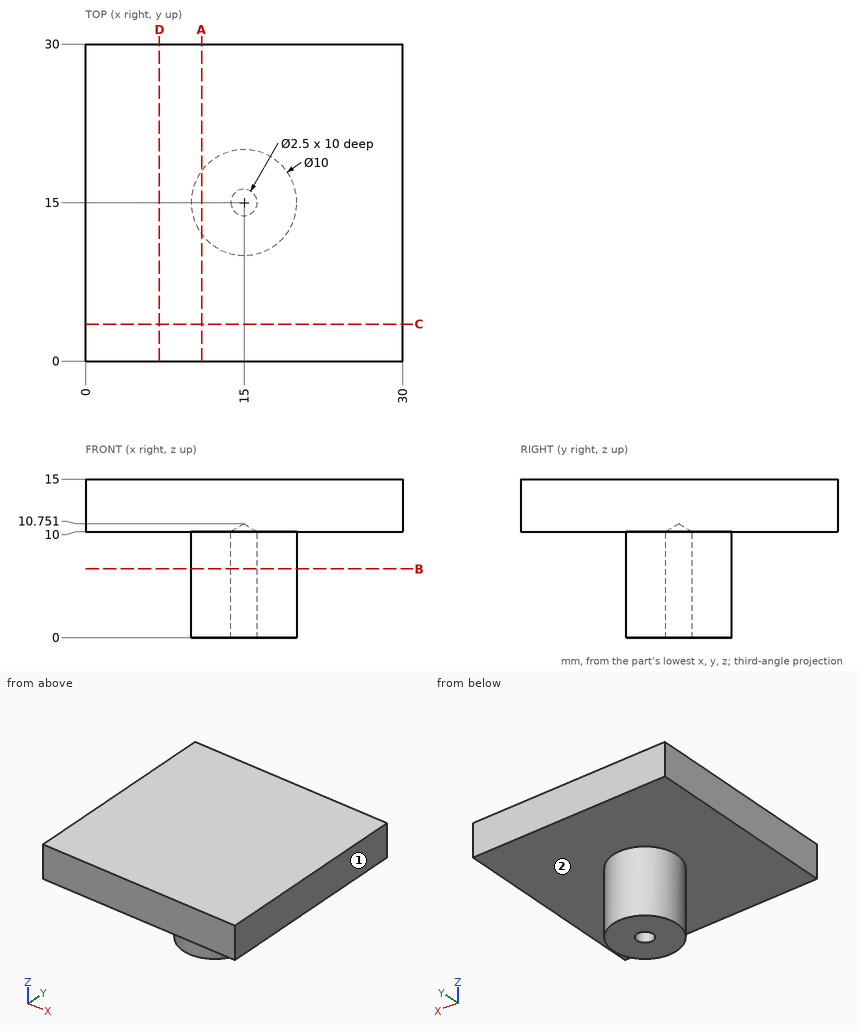
Job drawing, mm, ordinate dimensions from the low corner. One solid piece. A direction names the side the tool comes from. Coordinates: 2 decimals unless noted, no trailing zeros. Write each loop counter-clockwise with the first axis right and the second up, starting at its lowest first coordinate (ties: lowest second). Pieces come first, ordered by that corner, then holes. Notation, with made-up numbers: M -31,4 L -4,4 A20 cw -4,24 Z; hole C 86.5,3.5 d9. An arc over 180 degrees is marked long. Answer as a JSON object with one key per item and string values. Group by question number.
1) Saw through at A-A (x = 11). Write the cut outline in (y, z).
2) Pin check, flat tips, straight feed: pin 1 Ø1.5 at (y, z) = (3, 7.5) entering from -X; pin 2 Ø3 at (x, z) = (26.5, 12.5) entering from -Y; pin 3 Ø3 at (y, z) = (10.5, 7.5) entering from -X; pin 4 Ø2 at (x, y) = (15, 15) entering from -Z. Stop position of each tip, or through.
3) Tool access for the marked faces 1 and 2: list every direction of +Z, -Z, +X, -X, +Y, -Y with a clear straight run to the whole face (end or side of a thin tool).
4) Saw through at B-B (z = 6.5). Write the cut outline in (x, y), plus the area to 3 significant figures.
5) Saw through at C-C (y = 3.5). Write the cut outline in (x, z), plus the area to 3 significant figures.
6) Wall check: line 1 (Y direction, x = 15, z = 3.5); line 2 (Z direction, x = 26.5, y = 20.25). Give the ranges that are in metal, low to high. Write a range as from..to.
Values follow:
{
 "1": {"outline": "M 0,10 L 12,10 L 12,0 L 18,0 L 18,10 L 30,10 L 30,15 L 0,15 Z"},
 "2": {"pin 1": "passes through", "pin 2": "stops at y = 0", "pin 3": "stops at x = 11", "pin 4": "stops at z = 10.15"},
 "3": {"face 1": "+Z, -Z, +X, +Y, -Y", "face 2": "-Z"},
 "4": {"outline": "C 15,15 d10; hole C 15,15 d2.5", "area": "73.6 mm2"},
 "5": {"outline": "M 0,10 L 30,10 L 30,15 L 0,15 Z", "area": "150 mm2"},
 "6": {"line 1": "y = 10..13.75, 16.25..20", "line 2": "z = 10..15"}
}
